from build123d import *

# Parameters (mm, degrees)
F2_W     = 113.607649
F2_H     = 87.222615
F2_R     = 4.645393
F2_R_2   = 22.963932
F2_R_3   = 10.420251
F2_R_4   = 16.613932
F2_R_5   = 4.070252
F3_DEPTH = 2.54
F4_DEPTH = 13.335
F6_DEPTH = 2.54


with BuildPart() as f3:
    # F2 (on Front) → F3 (new body)
    with BuildSketch(Plane.XZ):
        with Locations((0.638156, 14.24115)):
            Rectangle(F2_W, F2_H)
        with Locations((-45.301553, -22.221763)):
            Circle(F2_R, mode=Mode.SUBTRACT)
        with Locations((-28.683275, 0)):
            Circle(F2_R_2, mode=Mode.SUBTRACT)
        with Locations((46.289496, -22.221763)):
            Circle(F2_R, mode=Mode.SUBTRACT)
        with Locations((28.683275, 0)):
            Circle(F2_R_2, mode=Mode.SUBTRACT)
        with Locations((0, 28.790265)):
            Circle(F2_R_3, mode=Mode.SUBTRACT)
        with Locations((-45.301553, 49.873423)):
            Circle(F2_R, mode=Mode.SUBTRACT)
        with Locations((45.644229, 49.873423)):
            Circle(F2_R, mode=Mode.SUBTRACT)
        with Locations((-28.683275, 0)):
            Circle(F2_R_2)
        with Locations((-28.683275, 0)):
            Circle(F2_R_4, mode=Mode.SUBTRACT)
        with Locations((0, 28.790265)):
            Circle(F2_R_3)
        with Locations((0, 28.790265)):
            Circle(F2_R_5, mode=Mode.SUBTRACT)
        with Locations((28.683275, 0)):
            Circle(F2_R_2)
        with Locations((28.683275, 0)):
            Circle(F2_R_4, mode=Mode.SUBTRACT)
    extrude(amount=F3_DEPTH)

    # F2 (on Front) → F4 (join)
    with BuildSketch(Plane.XZ):
        with Locations((0, 28.790265)):
            Circle(F2_R_3)
        with Locations((0, 28.790265)):
            Circle(F2_R_5, mode=Mode.SUBTRACT)
        with Locations((28.683275, 0)):
            Circle(F2_R_2)
        with Locations((28.683275, 0)):
            Circle(F2_R_4, mode=Mode.SUBTRACT)
        with Locations((-28.683275, 0)):
            Circle(F2_R_2)
        with Locations((-28.683275, 0)):
            Circle(F2_R_4, mode=Mode.SUBTRACT)
    extrude(amount=F4_DEPTH)

    # F5 (on face) → F6 (join)
    with BuildSketch(Plane(origin=(0, 0, 0), x_dir=(-1, 0, 0), z_dir=(0, 1, 0))):
        with BuildLine():
            Line((-12.350136, 3.041595), (-19.840281, 3.041595))
            Line((-19.840281, 3.041595), (-19.840281, -3.041595))
            Line((-19.840281, -3.041595), (-12.350136, -3.041595))
            ThreePointArc((-12.350136, -3.041595), (-12.069343, 0), (-12.350136, 3.041595))
        make_face()
        with BuildLine():
            Line((-37.526269, -3.041595), (-37.526269, 3.041595))
            Line((-37.526269, 3.041595), (-45.016414, 3.041595))
            ThreePointArc((-45.016414, 3.041595), (-45.297207, 0), (-45.016414, -3.041595))
            Line((-45.016414, -3.041595), (-37.526269, -3.041595))
        make_face()
        with BuildLine():
            Line((45.016414, 3.041595), (37.526269, 3.041595))
            Line((37.526269, 3.041595), (37.526269, -3.041595))
            Line((37.526269, -3.041595), (45.016414, -3.041595))
            ThreePointArc((45.016414, -3.041595), (45.297207, 0), (45.016414, 3.041595))
        make_face()
        with BuildLine():
            ThreePointArc((12.350136, 3.041595), (12.069343, 0), (12.350136, -3.041595))
            Line((12.350136, -3.041595), (19.840281, -3.041595))
            Line((19.840281, -3.041595), (19.840281, 3.041595))
            Line((19.840281, 3.041595), (12.350136, 3.041595))
        make_face()
    extrude(amount=-F6_DEPTH)


solid = f3.part
Source: CAD feature listing. Evaluate the final solid. Frame: model axes, mm. A direction names the side the tool comes from. Round coordinates to 2 decimals unless told otherwise and drop trailing zeros. Loops run counter-clockwise (first coordinate to the right, second up) from the corner with the lowest first, then second, coordinate; pieces in that order, holes last. Notation, with made-up numbers: (86, -16.5) -> (142, -16.5) arc R23 cw to (142, 21.5) -> close; hole circle Ø3 at (-33, -6). An arc over 180 degrees is marked (long way). Answer as a JSON object with one key per item and string values. Group by question number.
Q1. Section query C-C (y = -6.5). Output: boundary loops of the cut face in (x, z), plus the area to 3 significant figures.
Q2. Contact query for flat-ended pins moving along their axis: P1, Ø8, axis at y = -7, z = 37, coming from the +X side; P2, Ø5, axis at x = -9, z = 17, coming from the -Y side; P3, Ø5, axis at y = -6.5, z = -4, coming from the +X side. Output: stop coordinate, or through.
Q3. Section query A-A (x = 0). Output: boundary loops of the cut face in (y, z) (3 decimals), plus the area to 3 significant figures.
Q4. Section query B-B (z = 0). Output: boundary loops of the cut face in (x, y) (3 decimals).
Q5. Access query for faces 4 (the cylindrical face through (11.76, -7.86, 15.52)), 5 (the flat face through (-41, -1, 3.042)), 6 (the flat face through (44, -13.335, 7)). Directions: +Z, -Z, +X, -X, +Y, -Y. A direction counts if a zero-diameter tool reaches every point of the face in a straight line with its end or side. Return the directions, or none.
Q6. Mould query, pull axis Z, two halves, no side actions, for faces 1 (the flat face through (0, -1, 57.852)), 2 (the flat face through (4.5, -13.335, 28.9)), 3 (the cylindrical face through (-41.01, -1.25, -24)). Classes: pulls with the +Z half, pulls with the -Z half, needs draft (parallel to the pull), parting line crosses it, or undercut.
Q7. Section query D-D (x = 14.5). Output: boundary loops of the cut face in (y, z) (3 decimals).
Q8. Ray query, line 1 (Y direction, x = 27, z = 39); line 2 (X direction, y = -8.75, z = 7); line 3 (Z direction, x = 23.5, y = -6.5). Return the intervals inside material, ascending. Write a range as from..to.
Completed:
{
 "1": {"outline": "circle Ø45.93 at (-28.68, 0); circle Ø20.84 at (0, 28.79); circle Ø45.93 at (28.68, 0); hole circle Ø33.23 at (-28.68, 0); hole circle Ø8.14 at (0, 28.79); hole circle Ø33.23 at (28.68, 0)", "area": "1,870 mm²"},
 "2": {"P1": "x = 9.53", "P2": "y = -2.54", "P3": "x = 51.6"},
 "3": {"outline": "(-13.335, 18.37) -> (-2.54, 18.37) -> (-2.54, -29.37) -> (0, -29.37) -> (0, 24.72) -> (-13.335, 24.72) -> close; (-13.335, 32.861) -> (0, 32.861) -> (0, 57.852) -> (-2.54, 57.852) -> (-2.54, 39.211) -> (-13.335, 39.211) -> close", "area": "338 mm²"},
 "4": {"outline": "(-56.166, -2.54) -> (-51.647, -2.54) -> (-51.647, -13.335) -> (-45.297, -13.335) -> (-45.297, -2.54) -> (-37.526, -2.54) -> (-37.526, 0) -> (-56.166, 0) -> close; (-19.84, -2.54) -> (-12.069, -2.54) -> (-12.069, -13.335) -> (-5.719, -13.335) -> (-5.719, -2.54) -> (5.719, -2.54) -> (5.719, -13.335) -> (12.069, -13.335) -> (12.069, -2.54) -> (19.84, -2.54) -> (19.84, 0) -> (-19.84, 0) -> close; (37.526, -2.54) -> (45.297, -2.54) -> (45.297, -13.335) -> (51.647, -13.335) -> (51.647, -2.54) -> (57.442, -2.54) -> (57.442, 0) -> (37.526, 0) -> close"},
 "5": {"face 4": "-Y", "face 5": "+Y, -Y", "face 6": "+Z, -Z, +X, -X, -Y"},
 "6": {"face 1": "pulls with the +Z half", "face 2": "needs draft", "face 3": "undercut"},
 "7": {"outline": "(-13.335, -18.06) -> (-2.54, -18.06) -> (-2.54, -29.37) -> (0, -29.37) -> (0, -8.652) -> (-13.335, -8.652) -> close; (-13.335, 8.652) -> (0, 8.652) -> (0, 57.852) -> (-2.54, 57.852) -> (-2.54, 18.06) -> (-13.335, 18.06) -> close; (-2.54, -3.042) -> (0, -3.042) -> (0, 3.042) -> (-2.54, 3.042) -> close"},
 "8": {"line 1": "-2.54..0", "line 2": "-50.55..-43.75, -13.62..-6.81, 6.81..13.62, 43.75..50.55", "line 3": "-22.37..-15.78, 15.78..22.37"}
}
